Here's the drawing with two shaded views (mm, measured from the low corner). I have some questions. A direction names the side the tool comes from. Give positions to 0.01 mm unless a question says otherwise; leave off trailing zeros. Write each loop counter-clockwise with the first axis right and the second up, starting at its lowest first coordinate (ties: lowest second). Pieces come first, ordered by that corner, then holes. Notation, with made-up numbers: (24.25, 64.25) - (60.25, 64.25) arc R32 ccw to (60.25, 92.25) - close; hole circle Ø5 at (81.25, 82.25). An arc over 180 degrees is marked (long way). Answer as CSV lines item,"result". Start each with the question number.
Q1. Imagine slicing it at A-A on z = 23. List the corners of the cut face in (x, y) for me.
Q2. On a 3-axis mill with a long thin cutter (end or side, diameter ignored), from which of +Z, -Z, +X, -X, +Y, -Y can I reach the whole of each face in a straight line? I mean the marked faces 1, 2 and 3. Say none if no direction works.
Q3. We'd pull the mould along Z, two halves only. Please class the marked faces 4, 5, 6 and 7: pulls with the +Z half, pulls with the -Z half, needs draft (parallel to the pull), parting line crosses it, or undercut.
Q4. Imagine slicing it at B-B on x = 6. List the corners of the cut face in (y, z) for me, and give its area (3 significant figures).
Q5. Will these pins go through, and if not, where does the flat tip stop? pin 1 Ø8 at (x, z) = (11.5, 23) entering from +Y; pin 2 Ø7 at (y, z) = (8, 3) entering from -X; pin 3 Ø2 at (x, y) = (15, 11.5) entering from +Z.
Q6. Imagine slicing it at D-D on x = 15. List the corners of the cut face in (y, z) for me, and give its area (3 significant figures).
Q7. Imagine slicing it at C-C on z = 8. List the corners of the cut face in (x, y) for me, and give its area (3 significant figures).
Q8. If I drill on line 1 along X through (y, z) = (0.7, 23); line 2 along Y through (x, z) = (15, 5); line 3 along X through (y, z) = (4.75, 3.5), over which ranges is the centre line in solid material (lowest first)?
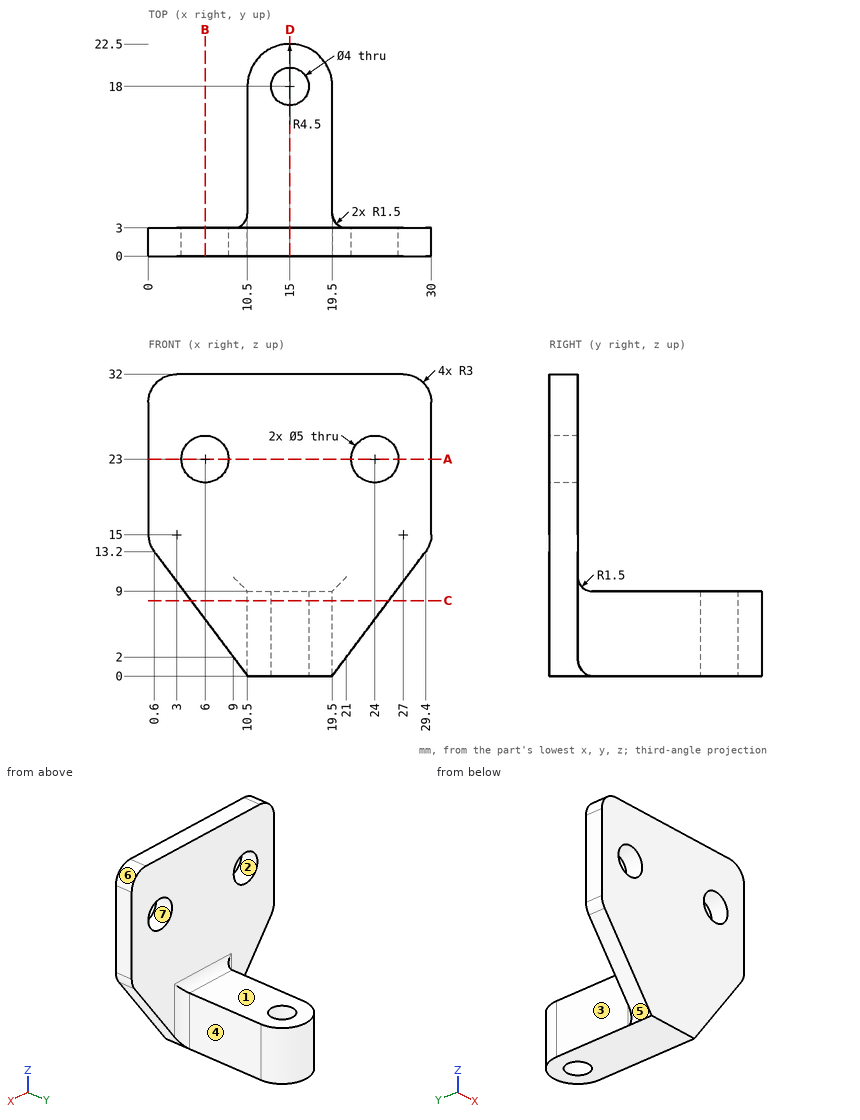
Conclusion:
1,outline,"(0, 0) - (3.5, 0) - (3.5, 3) - (0, 3) - close; (8.5, 0) - (21.5, 0) - (21.5, 3) - (8.5, 3) - close; (26.5, 0) - (30, 0) - (30, 3) - (26.5, 3) - close"
2,face 1,"+Z, +X, -X, +Y"
2,face 2,"+Y, -Y"
2,face 3,"+Z, -Z, -X, +Y"
3,face 4,"needs draft"
3,face 5,"pulls with the -Z half"
3,face 6,"pulls with the +Z half"
3,face 7,"undercut"
4,outline,"(0, 6) - (3, 6) - (3, 20.5) - (0, 20.5) - close; (0, 25.5) - (3, 25.5) - (3, 32) - (0, 32) - close"
4,area,"63.0 mm^2"
5,pin 1,"y = 3"
5,pin 2,"x = 10.5"
5,pin 3,"z = 9"
6,outline,"(0, 0) - (16, 0) - (16, 9) - (4.5, 9) arc R1.5 cw to (3, 10.5) - (3, 32) - (0, 32) - close; (20, 0) - (22.5, 0) - (22.5, 9) - (20, 9) - close"
6,area,"236 mm^2"
7,outline,"(4.5, 0) - (25.5, 0) - (25.5, 3) - (21, 3) arc R1.5 cw to (19.5, 4.5) - (19.5, 18) arc R4.5 ccw to (10.5, 18) - (10.5, 4.5) arc R1.5 cw to (9, 3) - (4.5, 3) - close; hole circle Ø4 at (15, 18)"
7,area,"218 mm^2"
8,line 1,"0 to 3.5, 8.5 to 21.5, 26.5 to 30"
8,line 2,"0 to 16, 20 to 22.5"
8,line 3,"10.5 to 19.5"
